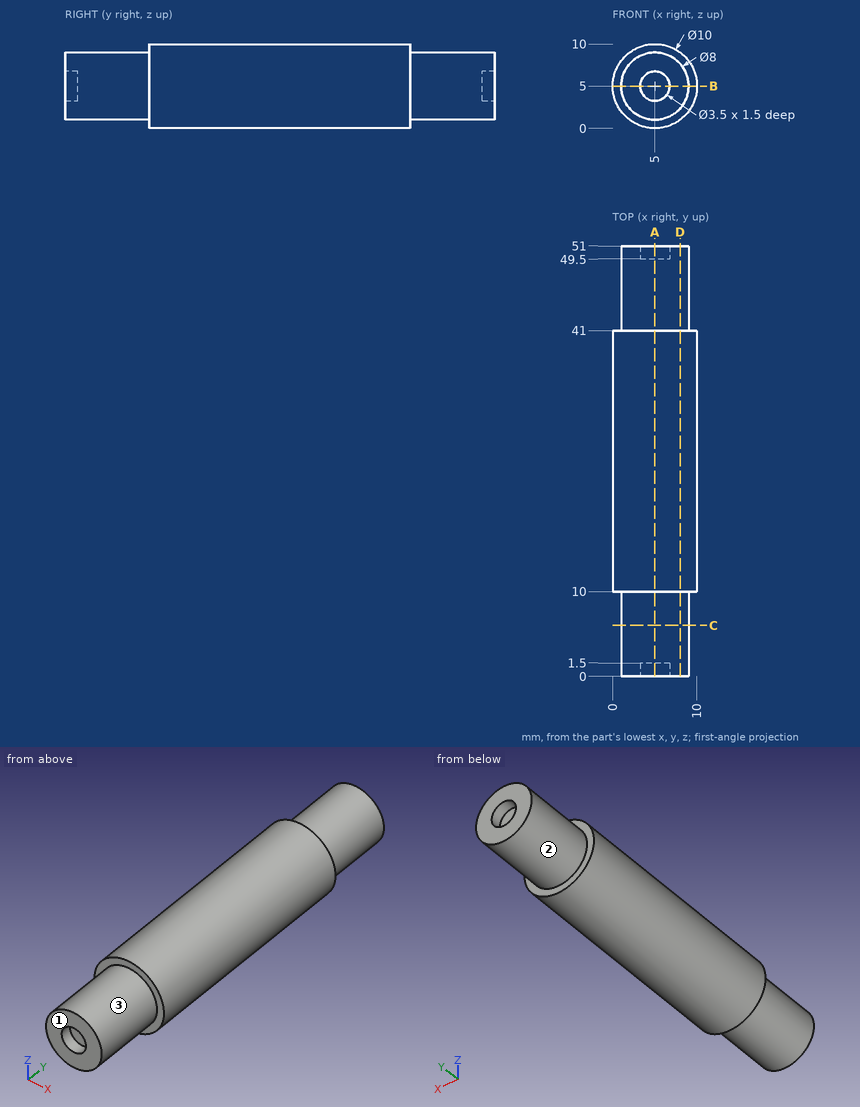
Verification items for this drawing (mm, ordinates from the low corner). A direction names the side the tool comes from. Give positions to 0.01 mm unless a question says otherwise; leave off trailing zeros. Order: outer loops, then holes, each group sorted by start corner. A loop starts at its lowest first (then second) coordinate and runs counter-clockwise, first axis right, second up.
1) Tool access check on the marked faces 1, 2 and 3. Record the directions out of +Z, -Z, +X, -X, +Y, -Y that give a thin tool (end or side, any length) a straight path to the whole face; none if there is none.
Results are:
face 1: +Z, -Z, +X, -X, -Y
face 2: +Y
face 3: -Y
2) Cross-section at C-C (y = 6). Record the boundary of the cut face in (x, z).
Results are:
outline: circle Ø8 at (5, 5)
3) Cross-section at A-A (x = 5). Record the boundary of the cut face in (y, z), then the cut area to 4 significant figures.
Results are:
outline: (0, 1) - (10, 1) - (10, 0) - (41, 0) - (41, 1) - (51, 1) - (51, 3.25) - (49.5, 3.25) - (49.5, 6.75) - (51, 6.75) - (51, 9) - (41, 9) - (41, 10) - (10, 10) - (10, 9) - (0, 9) - (0, 6.75) - (1.5, 6.75) - (1.5, 3.25) - (0, 3.25) - close
area: 459.5 mm2
4) Cross-section at B-B (z = 5). Record the boundary of the cut face in (x, y).
Results are:
outline: (0, 10) - (1, 10) - (1, 0) - (3.25, 0) - (3.25, 1.5) - (6.75, 1.5) - (6.75, 0) - (9, 0) - (9, 10) - (10, 10) - (10, 41) - (9, 41) - (9, 51) - (6.75, 51) - (6.75, 49.5) - (3.25, 49.5) - (3.25, 51) - (1, 51) - (1, 41) - (0, 41) - close
5) Cross-section at D-D (x = 8). Record the boundary of the cut face in (y, z).
Results are:
outline: (0, 2.35) - (10, 2.35) - (10, 1) - (41, 1) - (41, 2.35) - (51, 2.35) - (51, 7.65) - (41, 7.65) - (41, 9) - (10, 9) - (10, 7.65) - (0, 7.65) - close
6) Material ranges on probe 1 along X at (y, z) = (49.9, 5); probe 2 along Z at (x, y) = (4.75, 14), recorded low to high.
Results are:
probe 1: x = 1 to 3.25, 6.75 to 9
probe 2: z = 0.01 to 9.99
7) Gauge pin test, flat ends, axial feed: pin 1 (4 mm diameter, centred on x = 5, z = 5, fed in from -Y); pin 2 (1.5 mm diameter, centred on y = 33.5, z = 8, fed in from +X). Record the tip position at first contact, or that the pin passes through.
Results are:
pin 1: stops at y = 0
pin 2: stops at x = 9.47
